from build123d import *

# Parameters (mm, degrees)
F0_W     = 38.1
F0_H     = 6.35
F1_DEPTH = 10.16
F2_R     = 6.34999
F4_DEPTH = 25.4


# Not quite as in the source:
# - a fillet or chamfer is up to 0.001 mm smaller than in the source, because OpenCascade refuses the exact size


with BuildPart() as f1:
    # F0 (on Top) → F1 (new body)
    with BuildSketch(Plane.XY):
        with Locations((0, 3.175)):
            Rectangle(F0_W, F0_H)
    extrude(amount=F1_DEPTH)

    # F2 (radius 6.35 in the source; OpenCascade refuses exactly that, so slightly less here)
    f2_edges = [f1.edges().sort_by_distance(p)[0] for p in [
        (0, 6.35, 10.16),
    ]]
    fillet(f2_edges, radius=F2_R)

    # F3 (on face) → F4 (cut)
    with BuildSketch(Plane.XZ):
        with BuildLine():
            ThreePointArc((-16.637, 10.16), (-15.24, 8.763), (-13.843, 10.16))
            Line((-13.843, 10.16), (-16.637, 10.16))
        make_face()
        with BuildLine():
            Line((-3.8735, 10.16), (-6.2865, 10.16))
            ThreePointArc((-6.2865, 10.16), (-5.08, 8.9535), (-3.8735, 10.16))
        make_face()
        with BuildLine():
            Line((5.9055, 10.16), (4.2545, 10.16))
            ThreePointArc((4.2545, 10.16), (5.08, 9.3345), (5.9055, 10.16))
        make_face()
        with BuildLine():
            Line((15.875, 10.16), (14.605, 10.16))
            ThreePointArc((14.605, 10.16), (15.24, 9.525), (15.875, 10.16))
        make_face()
    extrude(amount=-F4_DEPTH, mode=Mode.SUBTRACT)


solid = f1.part
Could you check a few things on this model? Use its own coordinates, in mm. Round coordinates to 2 decimals unless told otherwise and drop trailing zeros. Write each loop counter-clockwise with the first axis right and the second up, starting at its lowest first coordinate (ties: lowest second). Pieces come first, ordered by that corner, then holes. Notation, with made-up numbers: (-27.5, 52) - (-15.5, 52) arc R25 cw to (-15.5, 67) - close; hole circle Ø4 at (-15, 63.25). An arc over 180 degrees is marked (long way). Put each result on its own line as item: value. Start each with the question number.
(1) I want a section at C-C, the plane z = 7.75. Please give me the cut outline in (x, y).
(2) Will these pins go through, and if not, where does the flat tip stop? pin 1 (1.5 mm diameter, centred on x = 14, y = 4, fed in from +Z); pin 2 (2 mm diameter, centred on x = 8.5, y = 3, fed in from +Z).
(3) Thinking about a two-plate mould opening in X: for faces 1 (the flat face through (0, 6.35, 2)), 2 (the cylindrical face through (-5.107, 1.422, 8.954)), 3 (the flat face through (19.05, 3, 5)), which applies, released by +X, released by -X, zero draft, split by the parting line, or undercut?
(4) I need wall thicknesses on probe 1 along Z at (x, y) = (-6.5, 4); probe 2 along Y at (x, z) = (13, 5.25); probe 3 along Z at (x, y) = (-9, 3). Which ranges of each line are inside material? Lowest first, please.
(5) I want a section at A-A, the plane x = -15.24. Please give me the cut outline in (y, z), plus the area to 3 significant figures.
Here are the results:
1. outline: (-19.05, 0) - (19.05, 0) - (19.05, 4.98) - (-19.05, 4.98) - close
2. pin 1: stops at z = 9.27
2. pin 2: stops at z = 9.84
3. face 1: zero draft
3. face 2: undercut
3. face 3: released by +X
4. probe 1: z = 0 to 8.74
4. probe 2: y = 0 to 6.18
4. probe 3: z = 0 to 9.41
5. outline: (0, 0) - (6.35, 0) - (6.35, 3.81) arc R6.35 ccw to (3.97, 8.76) - (0, 8.76) - close
5. area: 52.1 mm^2
